Verification items for the finished model (mm, model axes). Face numbers are marked on the shaded views. A direction names the side the tool comes from. Round coordinates to 2 decimals unless told otherwise and drop trailing zeros. Write each loop counter-clockwise with the first axis right and the second up, starting at its lowest first coordinate (ties: lowest second). Pieces come first, ordered by that corner, then holes. Notation, with made-up numbers: M 66,71.5 L 125,71.5 A10 ccw 125,90.5 Z; hole C -13,5.5 d10. An arc over 180 degrees is marked long. One line per question, with ' | ' between items. Start each with the question number.
Q1. Cross-section at B-B (z = 10). Record the boundary of the cut face in (x, y), then the cut area to 3 significant figures.
Q2. Thickness scan on line 1 along Z through (x, y) = (1, -67); line 2 along Y through (x, z) = (18, 19); line 3 along X through (y, z) = (-66.5, 5.5). Record the ranges inside material, lowest first. Write a range as from..to.
Q3. Cross-section at C-C (x = 94). Record the boundary of the cut face in (y, z), then the cut area to 3 significant figures.
Q4. Cross-section at A-A (y = -67). Record the boundary of the cut face in (x, z).
Q5. Cross-section at D-D (y = -53). Record the boundary of the cut face in (x, z).
Q6. Tool access check on the marked faces 1, 2 and 3. Record the directions out of +Z, -Z, +X, -X, +Y, -Y that give a thin tool (end or side, any length) a straight path to the whole face; none if there is none.
Q7. Gauge pin test, flat ends, axial feed: pin 1 (3 mm diameter, centred on x = 53, y = -15, fed in from +Z); pin 2 (12 mm diameter, centred on x = 84, z = 41.5, fed in from -Y); pin 3 (3.5 mm diameter, centred on x = 61.5, y = -58.5, fed in from +Z). Record the tip position at first contact, or that the pin passes through.
from build123d import *

# Parameters (mm, degrees)
CYLINDER_R            = 2
CYLINDER_DEPTH        = 10
FUSION002_PITCH_ANGLE = 90
FUSION001_PITCH_ANGLE = 90
BOX004_W              = 10
BOX004_H              = 10
BOX004_DEPTH          = 10
BOX003_W              = 70
BOX003_H              = 10
BOX003_DEPTH          = 10
FILLET_R              = 3
BOX001_W              = 112
BOX001_H              = 53
BOX001_DEPTH          = 57
BOX_W                 = 115
BOX_H                 = 56
BOX_DEPTH             = 60
BOX002_W              = 5
BOX002_H              = 56
BOX002_DEPTH          = 15
FILLET001_R           = 3
CUT004_ROLL_ANGLE     = 90


with BuildPart() as cone:
    # Cone → Cone (revolve)
    with BuildSketch(Plane(origin=(0, 0, 10), x_dir=(1, 0, 0), z_dir=(0, -1, 0))):
        Polygon((0, 0), (2, 0), (4, 2), (0, 2), align=None)
    revolve(axis=Axis((0, 0, 10), (0, 0, 1)))


with BuildPart() as cylinder:
    # Cylinder → Cylinder (new body)
    with BuildSketch(Plane.XY):
        Circle(CYLINDER_R)
    extrude(amount=CYLINDER_DEPTH)


with BuildPart() as screw_cutout001:
    # Fusion002 base: copy of Cylinder
    add(cylinder.part)

    # Fusion002: union Cone
    add(cone.part)


with BuildPart() as screw_cutout001_1:
    # Fusion002 pitch: moved
    add(screw_cutout001.part.rotate(Axis((0, 0, 0), (0, 1, 0)), FUSION002_PITCH_ANGLE))


with BuildPart() as screw_cutout001_2:
    # Fusion002 placement: moved
    add(screw_cutout001_1.part.moved(Location((-7, 10, 67))))


with BuildPart() as fusion003:
    # Fusion001 base: copy of Cylinder
    add(cylinder.part)

    # Fusion001: union Cone
    add(cone.part)


with BuildPart() as fusion003_1:
    # Fusion001 pitch: moved
    add(fusion003.part.rotate(Axis((0, 0, 0), (0, 1, 0)), FUSION001_PITCH_ANGLE))


with BuildPart() as fusion003_2:
    # Fusion001 placement: moved
    add(fusion003_1.part.moved(Location((-7, 46, 67))))

    # Fusion003: union screw cutout001
    add(screw_cutout001_2.part)


with BuildPart() as cablecutout001:
    # Box004 → Box004 (new body)
    with BuildSketch(Plane(origin=(75, 46, 51), x_dir=(1, 0, 0), z_dir=(0, 0, 1))):
        with Locations((5, 5)):
            Rectangle(BOX004_W, BOX004_H)
    extrude(amount=BOX004_DEPTH)


with BuildPart() as fillet_body:
    # Box003 → Box003 (new body)
    with BuildSketch(Plane(origin=(30, 46, 51), x_dir=(1, 0, 0), z_dir=(0, 0, 1))):
        with Locations((35, 5)):
            Rectangle(BOX003_W, BOX003_H)
    extrude(amount=BOX003_DEPTH)

    # Cut002: cut cablecutout001
    add(cablecutout001.part, mode=Mode.SUBTRACT)

    # Fillet
    fillet_edges = [fillet_body.edges().sort_by_distance(p)[0] for p in [
        (30, 46, 56),
        (75, 46, 56),
        (100, 46, 56),
        (85, 46, 56),
    ]]
    fillet(fillet_edges, radius=FILLET_R)


with BuildPart() as cube001:
    # Box001 → Box001 (new body)
    with BuildSketch(Plane(origin=(0, 3, 0), x_dir=(1, 0, 0), z_dir=(0, 0, 1))):
        with Locations((56, 26.5)):
            Rectangle(BOX001_W, BOX001_H)
    extrude(amount=BOX001_DEPTH)


with BuildPart() as cut:
    # Box → Box (new body)
    with BuildSketch(Plane.XY):
        with Locations((57.5, 28)):
            Rectangle(BOX_W, BOX_H)
    extrude(amount=BOX_DEPTH)

    # Cut: cut Cube001
    add(cube001.part, mode=Mode.SUBTRACT)


with BuildPart() as cut004:
    # Box002 → Box002 (new body)
    with BuildSketch(Plane.XY.offset(60)):
        with Locations((2.5, 28)):
            Rectangle(BOX002_W, BOX002_H)
    extrude(amount=BOX002_DEPTH)

    # Fillet001
    fillet001_edges = [cut004.edges().sort_by_distance(p)[0] for p in [
        (2.5, 0, 75),
        (2.5, 56, 75),
    ]]
    fillet(fillet001_edges, radius=FILLET001_R)

    # Fusion: union Cut
    add(cut.part)

    # Cut003: cut Fillet body
    add(fillet_body.part, mode=Mode.SUBTRACT)

    # Cut004: cut Fusion003
    add(fusion003_2.part, mode=Mode.SUBTRACT)


with BuildPart() as cut004_1:
    # Cut004 roll: moved
    add(cut004.part.rotate(Axis((0, 0, 0), (1, 0, 0)), CUT004_ROLL_ANGLE))


with BuildPart() as cut004_2:
    # Cut004 placement: moved
    add(cut004_1.part)


solid = cut004_2.part
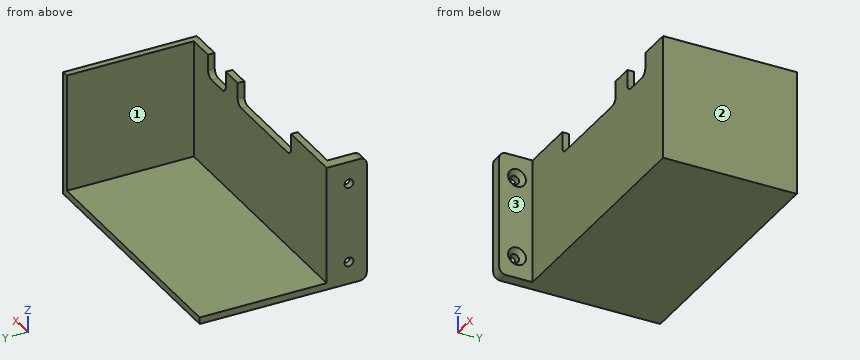
Determined:
1) outline: M 0,-75 L 5,-75 L 5,-71 L 3,-69 L 0,-69 Z; M 0,-65 L 3,-65 L 5,-63 L 5,-60 L 115,-60 L 115,0 L 112,0 L 112,-57 L 0,-57 Z | area: 567 mm²
2) line 1: z = 0..8, 12..44, 48..56 | line 2: y = -60..-57 | line 3: x = 0..5
3) outline: M -60,0 L 0,0 L 0,3 L -57,3 L -57,46 L -60,46 Z | area: 309 mm²
4) outline: M 0,0 L 5,0 L 5,6 L 3,8 L 0,8 Z; M 0,12 L 3,12 L 5,14 L 5,42 L 3,44 L 0,44 Z; M 0,48 L 3,48 L 5,50 L 5,56 L 0,56 Z
5) outline: M 0,0 L 115,0 L 115,56 L 112,56 L 112,3 L 0,3 Z
6) face 1: +Z, -X, +Y | face 2: +Z, -Z, +X, +Y, -Y | face 3: +Z, -Z, +X, -Y
7) pin 1: stops at z = 3 | pin 2: stops at y = -60 | pin 3: stops at z = 46
